Build history of the part. All positions in model axes, mm. Face numbers are marked on the shaded views. A direction names the side the tool comes from. Coordinates: 2 decimals unless noted, no trailing zeros. Order: outer loops, then holes, each group sorted by start corner. A loop starts at its lowest first (then second) coordinate and runs counter-clockwise, first axis right, second up. Notation, with made-up numbers: (73.5, 15.5) -> (98.5, 15.5) arc R29 cw to (98.5, 40.5) -> close; hole circle Ø10 at (-38.75, 6). An arc over 180 degrees is marked (long way). Write each question's results on one line, items separated by ' | '.
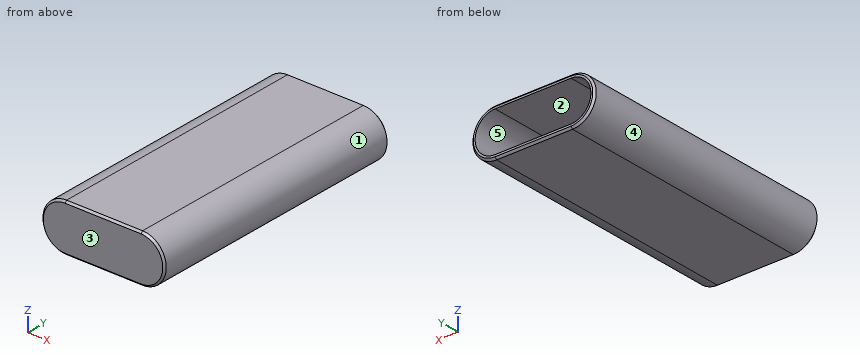
from build123d import *

# Parameters (mm, degrees)
SKETCH2_W               = 14.9
SKETCH2_H               = 11.7
SKETCH2_W_2             = 8.7
SKETCH2_H_2             = 7.7
BOSS_EXTRUDE1_DEPTH     = 12.6
CUT_EXTRUDE1_DEPTH      = 16.288067242
CUT_EXTRUDE1_DEPTH_BACK = 16.288067242
SKETCH4_W               = 4.6
SKETCH4_H               = 3.25
BOSS_EXTRUDE2_DEPTH     = 3
BOSS_EXTRUDE3_START     = 137
BOSS_EXTRUDE3_DEPTH     = 137
CHAMFER1_SIZE           = 1
CHAMFER2_SIZE           = 0.8
CHAMFER3_SIZE           = 2


with BuildPart() as part:
    # Sketch2 → Boss-Extrude1 (new body)
    with BuildSketch(Plane.XZ.offset(-12)):
        Rectangle(SKETCH2_W, SKETCH2_H)
        Rectangle(SKETCH2_W_2, SKETCH2_H_2, mode=Mode.SUBTRACT)
    extrude(amount=BOSS_EXTRUDE1_DEPTH)

    # Sketch4 → Cut-Extrude1 (cut, two sides: drawn at the far end of the back side and taken through both)
    with BuildSketch(Plane(origin=(0, 0, 0), x_dir=(0, 0, -1), z_dir=(1, 0, 0)).offset(-CUT_EXTRUDE1_DEPTH_BACK)):
        with Locations((0, 8.625)):
            Rectangle(SKETCH4_W, SKETCH4_H)
    extrude(amount=CUT_EXTRUDE1_DEPTH + CUT_EXTRUDE1_DEPTH_BACK, mode=Mode.SUBTRACT)

    # Sketch5 → Boss-Extrude2 (add)
    with BuildSketch(Plane.XZ.offset(0.6)):
        with BuildLine():
            Line((-20, 12.5), (20, 12.5))
            ThreePointArc((20, 12.5), (32.5, 0), (20, -12.5))
            Line((20, -12.5), (-20, -12.5))
            ThreePointArc((-20, -12.5), (-32.5, 0), (-20, 12.5))
        make_face()
    extrude(amount=BOSS_EXTRUDE2_DEPTH)

    # Sketch7 → Boss-Extrude3 (add)
    with BuildSketch(Plane(origin=(0, -0.6, 0), x_dir=(1, 0, 0), z_dir=(0, 1, 0)).offset(BOSS_EXTRUDE3_START)):
        with BuildLine():
            Line((-20, -12.5), (20, -12.5))
            ThreePointArc((20, -12.5), (32.5, 0), (20, 12.5))
            Line((20, 12.5), (-20, 12.5))
            ThreePointArc((-20, 12.5), (-32.5, 0), (-20, -12.5))
        make_face()
        with BuildLine():
            Line((-20, -10.5), (20, -10.5))
            ThreePointArc((20, -10.5), (30.5, 0), (20, 10.5))
            Line((20, 10.5), (-20, 10.5))
            ThreePointArc((-20, 10.5), (-30.5, 0), (-20, -10.5))
        make_face(mode=Mode.SUBTRACT)
    extrude(amount=-BOSS_EXTRUDE3_DEPTH)

    # Chamfer1
    chamfer1_edges = [part.edges().sort_by_distance(p)[0] for p in [
        (-32.5, -3.6, 0),
        (0, -3.6, -12.5),
        (32.5, -3.6, 0),
        (0, -3.6, 12.5),
        (-32.5, 136.4, 0),
        (0, 136.4, 12.5),
        (32.5, 136.4, 0),
        (0, 136.4, -12.5),
    ]]
    chamfer(chamfer1_edges, length=CHAMFER1_SIZE)

    # Chamfer2
    chamfer2_edges = [part.edges().sort_by_distance(p)[0] for p in [
        (0, 12, -3.85),
        (4.35, 12, 0),
        (0, 12, 3.85),
        (-4.35, 12, 0),
        (0, 12, -5.85),
        (-7.45, 12, 0),
        (0, 12, 5.85),
        (7.45, 12, 0),
    ]]
    chamfer(chamfer2_edges, length=CHAMFER2_SIZE)

    # Chamfer3
    # the kernel refuses this chamfer: 2 mm, written as the material it takes off along each edge
    with BuildSketch(Plane(origin=(-7.45, 16.343365976, 5.85), x_dir=(-0.027495876610586053, 0, -0.9996219169112968), z_dir=(0, -1, 0)), Plane(origin=(7.45, 16.343365976, 5.85), x_dir=(-0.9996219169112968, 0, 0.027495876610586487), z_dir=(0, -1, 0))) as chamfer3_piece_1:
        Polygon((CHAMFER3_SIZE * 0.999621916911, CHAMFER3_SIZE * 0.0274958766106), (-CHAMFER3_SIZE * 0.0274958766106, CHAMFER3_SIZE * 0.999621916911), (0, 0), align=None)
    extrude(amount=16.943365976, mode=Mode.SUBTRACT)
    with BuildSketch(Plane(origin=(-7.45, 16.343365976, -5.85), x_dir=(-0.027495876610586924, 0, 0.9996219169112968), z_dir=(0, -1, 0)), Plane(origin=(7.45, 16.343365976, -5.85), x_dir=(-0.9996219169112968, 0, -0.027495876610586487), z_dir=(0, -1, 0))) as chamfer3_piece_2:
        Polygon((CHAMFER3_SIZE * 0.999621916911, -CHAMFER3_SIZE * 0.0274958766106), (-CHAMFER3_SIZE * 0.0274958766106, -CHAMFER3_SIZE * 0.999621916911), (0, 0), align=None)
    extrude(amount=16.943365976, mode=Mode.SUBTRACT)


solid = part.part
Item 1: Drill centre lines: line 1 (Y direction, x = -10.5, z = 4.25); line 2 (X direction, y = 86, z = 0.25); line 3 (Z direction, x = 4.5, y = 85). Where is each one in solid material? Low to high. Write a range as from..to.
Answer:
line 1: y = -3.6..-0.6 | line 2: x = -32.5..-30.5, 30.5..32.5 | line 3: z = -12.5..-10.5, 10.5..12.5
Item 2: Slice it at C-C, the plane x = 15.5. List the corners of the cut face in (y, z), and give its area (3 significant figures).
Answer:
outline: (-3.6, -11.5) -> (-2.6, -12.5) -> (135.4, -12.5) -> (136.4, -11.5) -> (136.4, -10.5) -> (-0.6, -10.5) -> (-0.6, 10.5) -> (136.4, 10.5) -> (136.4, 11.5) -> (135.4, 12.5) -> (-2.6, 12.5) -> (-3.6, 11.5) -> close | area: 621 mm^2
Item 3: Slice it at B-B, the plane y = 63. List the corners of the cut face in (x, z).
Answer:
outline: (-20, -12.5) -> (20, -12.5) arc R12.5 ccw to (20, 12.5) -> (-20, 12.5) arc R12.5 ccw to start; hole (-20, -10.5) -> (20, -10.5) arc R10.5 ccw to (20, 10.5) -> (-20, 10.5) arc R10.5 ccw to start
Item 4: Pin check, flat tips, straight feed: pin 1 (8 mm diameter, centred on y = 64, z = -3.5, fed in from -X); pin 2 (3.5 mm diameter, centred on x = 6.5, z = -1, fed in from +Y); pin 3 (8 mm diameter, centred on y = 49, z = -7, fed in from -X); pin 4 (2.5 mm diameter, centred on x = 2, z = 1.5, fed in from +Y). Stop position of each tip, or through.
Answer:
pin 1: stops at x = -32.5 | pin 2: stops at y = 12 | pin 3: stops at x = -32.13 | pin 4: stops at y = -0.6
Item 5: Slice it at A-A, the plane z = 0. State how many separate pieces and enclosed holes the cut face has, and give its area (3 significant figures).
Answer:
separate pieces: 3 | enclosed holes: 0 | area: 798 mm^2
Item 6: Pull direction X, two halves, no side cores. Call the marked faces 3, 4 and 5: released by +X, released by -X, zero draft, split by the parting line, or undercut.
Answer:
face 3: zero draft | face 4: released by -X | face 5: undercut
Item 7: Tool access for the marked faces 1 and 2: list every direction of +Z, -Z, +X, -X, +Y, -Y with a clear straight run to the whole face (end or side of a thin tool).
Answer:
face 1: +X, +Y, -Y | face 2: +Y
